Geometry: final body of the model. Coordinates: model frame, mm. A direction names the side the tool comes from. Give positions to 0.01 mm unless a question says otherwise; leave off trailing zeros. Write each loop counter-clockwise with the first axis right and the second up, starting at its lowest first coordinate (ties: lowest second). Pieces come first, ordered by that corner, then holes. Notation, with made-up numbers: M 43.5,60 L 53.5,60 A34 ccw 53.5,91 Z; hole C 69.25,-38 d4. An arc over 180 degrees is marked long. One line per question, with ' | ' between items.
from build123d import *

# Parameters (mm, degrees)
F1_DEPTH = 12.7
F2_W     = 12.7
F2_H     = 12.7
F3_DEPTH = 12.7


with BuildPart() as f1:
    # F0 (on Top) → F1 (new body)
    with BuildSketch(Plane.XY):
        Polygon((-40.525064, 35.351565), (-40.525064, -40.848435), (-27.825064, -40.848435), (-27.825064, 22.651565), (-2.425064, 22.651565), (-2.425064, -40.848435), (10.274936, -40.848435), (10.274936, 35.351565), align=None)
    extrude(amount=F1_DEPTH)

    # F2 (on face) → F3 (join)
    with BuildSketch(Plane.XY.offset(12.7)):
        with Locations((-34.175064, 3.601565)):
            Rectangle(F2_W, F2_H)
        with Locations((-34.175064, 29.001565)):
            Rectangle(F2_W, F2_H)
        with Locations((3.924936, 29.001565)):
            Rectangle(F2_W, F2_H)
        with Locations((3.924936, 3.601565)):
            Rectangle(F2_W, F2_H)
    extrude(amount=F3_DEPTH)


solid = f1.part
(1) Draft query along X for faces 4 (the face through (-2.425, -9, 10)), 5 (the face through (10.275, -3, 10)), 6 (the face through (-15, 35.352, 10)). Return one class per face: released by +X, released by -X, zero draft, split by the parting line, or undercut.
Working result:
face 4: undercut | face 5: released by +X | face 6: zero draft
(2) Cut plane C-C, the plane y = 30.5. Return loops of the section in (x, z).
Working result:
outline: M -40.53,0 L 10.27,0 L 10.27,25.4 L -2.43,25.4 L -2.43,12.7 L -27.83,12.7 L -27.83,25.4 L -40.53,25.4 Z
(3) Cut plane A-A, the plane z = 23. Return loops of the section in (x, y).
Working result:
outline: M -40.53,-2.75 L -27.83,-2.75 L -27.83,9.95 L -40.53,9.95 Z; M -40.53,22.65 L -27.83,22.65 L -27.83,35.35 L -40.53,35.35 Z; M -2.43,-2.75 L 10.27,-2.75 L 10.27,9.95 L -2.43,9.95 Z; M -2.43,22.65 L 10.27,22.65 L 10.27,35.35 L -2.43,35.35 Z
(4) Set-up query: faces 1 (the face through (-34, 9.952, 19)), 2 (the face through (-15, 29, 12.7)), 3 (the face through (-27.825, -10, 10)). Return all of +Z, -Z, +X, -X, +Y, -Y with unobstructed straight access to the full face (end or side cutting, diameter ignored); none if empty.
Working result:
face 1: +Z, +X, -X | face 2: +Z, +Y, -Y | face 3: +Z, -Z, -Y
(5) Cut plane B-B, the plane y = -36. Return loops of the section in (x, z).
Working result:
outline: M -40.53,0 L -27.83,0 L -27.83,12.7 L -40.53,12.7 Z; M -2.43,0 L 10.27,0 L 10.27,12.7 L -2.43,12.7 Z
(6) First-contact query: P1, Ø10, axis at x = -37.5, y = -26, coming from the +Z side; P2, Ø6.5, axis at x = 2, z = 21, coming from the -Y side; P3, Ø10, axis at x = -16.5, z = 6, coming from the -Y side. Flat tips, straight axial feed; report the tip coordinate or a pass-through.
Working result:
P1: stops at z = 12.7 | P2: stops at y = -2.75 | P3: stops at y = 22.65
(7) Cut plane D-D, the plane x = 2. Return loops of the section in (y, z).
Working result:
outline: M -40.85,0 L 35.35,0 L 35.35,25.4 L 22.65,25.4 L 22.65,12.7 L 9.95,12.7 L 9.95,25.4 L -2.75,25.4 L -2.75,12.7 L -40.85,12.7 Z
(8) Material intervals for L1, parallel to Y at x = -38, z = 14; L2, parallel to X at y = 9, z = 12.5; L3, parallel to Z at x = -13, y = 27, sorted ascending. Write a range as [from, to].
Working result:
L1: y = [-2.75, 9.95], [22.65, 35.35] | L2: x = [-40.53, -27.83], [-2.43, 10.27] | L3: z = [0, 12.7]
